from build123d import *

# Parameters (mm, degrees)
SKETCH2_R          = 1
CUT_EXTRUDE2_DEPTH = 12.020949889


with BuildPart() as part:
    # Sketch1 → Revolve1 (revolve)
    with BuildSketch(Plane.XY, mode=Mode.PRIVATE) as revolve1_sk:
        with BuildLine():
            add(Edge.make_bspline(
                [(1.901469747, -4.187890833), (3.997803393, -5.505352851), (2.40138715, -6.003675185), (0.316595481, -6.158045679)],
                knots=[0, 0, 0, 0, 1, 1, 1, 1], degree=3))
            Line((1.901469747, -4.187890833), (1.901469747, 1.312109167))
            Line((1.901469747, 1.312109167), (3.270835138, 1.312109167))
            ThreePointArc((3.270835138, 1.312109167), (3.457066196, 1.693980285), (3.356353959, 2.106732757))
            ThreePointArc((3.356353959, 2.106732757), (3.314000681, 2.158555901), (3.270835138, 2.209704452))
            ThreePointArc((3.270835138, 2.209704452), (1.788504548, 3.318079362), (-0.024669059, 3.689832486))
            Line((-0.024669059, 3.689832486), (-0.024669059, -6.158045679))
            Line((-0.024669059, -6.158045679), (0.316595481, -6.158045679))
        make_face()
    revolve(revolve1_sk.sketch.rotate(Axis((-0.024669059, -4.1454e-05, 0), (0, -1, 0)), 180), axis=Axis((-0.024669059, -4.1454e-05, 0), (0, -1, 0)))

    # Sketch2 → Cut-Extrude2 (cut, through all)
    with BuildSketch(Plane(origin=(0, -6.158045679, 0), x_dir=(-1, 0, 0), z_dir=(0, -1, 0))):
        with Locations(Location((0.024669059, 0, 0), (0, 0, 180))):
            Circle(SKETCH2_R)
    extrude(amount=-CUT_EXTRUDE2_DEPTH, mode=Mode.SUBTRACT)


solid = part.part
Check sheet for the modelled part. Datum: model origin and axes. Units: mm. Give positions to 0.01 mm unless a question says otherwise; leave off trailing zeros. Write each loop counter-clockwise with the first axis right and the second up, starting at its lowest first coordinate (ties: lowest second). Pieces come first, ordered by that corner, then holes. Notation, with made-up numbers: (66, 28.5) -> (89, 28.5) arc R22 ccw to (89, 52.5) -> close; hole circle Ø11 at (-31, -31.5). An arc over 180 degrees is marked (long way). One line per item, written item: value. Start each with the question number.
Item 1: Section check A-A on y = -1.5. Record the cut outline in (x, z).
Item 2: Draft check along Y on faces 1 (the cylindrical face through (1.504, -1.399, 1.172)), 2 (the cylindrical face through (0, -1, -1)). Enter one of: +Y half, -Y half, draft (parallel to the pull), parting line (faces both ways), or undercut.
Item 3: Material ranges on probe 1 along X at (y, z) = (-0.25, 0.5); probe 2 along Y at (x, z) = (-1.5, 2); probe 3 along Z at (x, y) = (-0.5, -3.5), recorded low to high. Write a range as from..to.
Item 4: Gauge pin test, flat ends, axial feed: pin 1 (4 mm diameter, centred on x = 2, y = -4, fed in from +Z); pin 2 (4 mm diameter, centred on y = -4, z = 2.5, fed in from -X); pin 3 (2 mm diameter, centred on y = -2, z = -2.5, fed in from +X). Record the tip position at first contact, or that the pin passes through.
Results list:
1. outline: circle Ø3.85 at (-0.02, 0); hole circle Ø2 at (-0.02, 0)
2. face 1: undercut
2. face 2: draft
3. probe 1: -1.88..-0.89, 0.84..1.84
3. probe 2: -5.74..-4.59, 1.31..2.94
3. probe 3: -1.87..-0.88, 0.88..1.87
4. pin 1: z = 2.88
4. pin 2: x = -2.79
4. pin 3: x = 1.18
